Model file for the job. Use its own axes, mm. Face numbers are marked on the shaded views. A direction names the side the tool comes from. Give positions to 0.01 mm unless a question says otherwise; leave off trailing zeros. Order: outer loops, then holes, each group sorted by start corner. A loop starts at its lowest first (then second) coordinate and runs counter-clockwise, first axis right, second up. Notation, with made-up numbers: (-3, 37) -> (13, 37) arc R20 ccw to (13, 76) -> close; hole circle Ø1 at (-19.5, 2). An arc over 180 degrees is marked (long way). Answer in a Markdown table with one row per item. Add a question column.
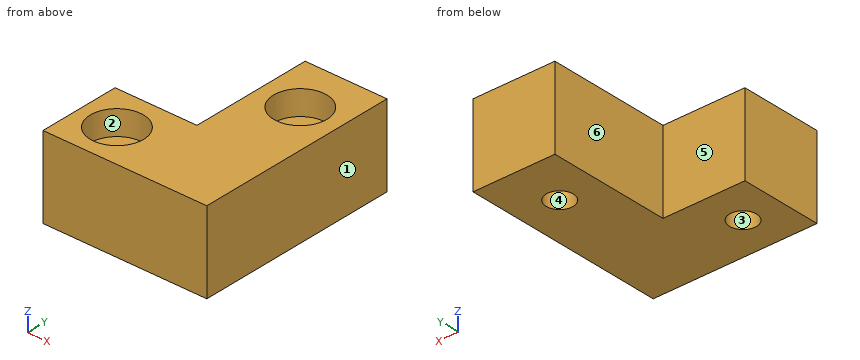
from build123d import *

# Parameters (mm, degrees)
F0_W           = 10
F0_H           = 10
F1_DEPTH       = 25
F2_W           = 10
F2_H           = 10
F3_DEPTH       = 10
F5_D           = 3.3
F5_CBORE_D     = 6.5
F5_CBORE_DEPTH = 3


with BuildPart() as f1:
    # F0 (on Front) → F1 (new body)
    with BuildSketch(Plane.XZ):
        Rectangle(F0_W, F0_H)
    extrude(amount=F1_DEPTH)

    # F2 (on face) → F3 (join)
    with BuildSketch(Plane(origin=(-5, 0, 0), x_dir=(0, -1, 0), z_dir=(-1, 0, 0))):
        with Locations((20, 0)):
            Rectangle(F2_W, F2_H)
    extrude(amount=F3_DEPTH)

    # F5 (through all)
    with Locations(Plane.XY.offset(5)):
        with Locations((0, -6.3472618349), (-10.296119377, -20.085208118)):
            CounterBoreHole(F5_D / 2, F5_CBORE_D / 2, F5_CBORE_DEPTH)


solid = f1.part
Item 1: Saw through at D-D on x = -13. List the corners of the cut face in (y, z).
Item 2: Pin check, flat tips, straight feed: pin 1 Ø12 at (x, y) = (-13, -21.5) entering from +Z; pin 2 Ø2 at (x, y) = (0, -6.35) entering from +Z; pin 3 Ø5 at (x, y) = (0, -6.35) entering from +Z; pin 4 Ø6 at (x, z) = (-9.5, -2.5) entering from +Y. Stop position of each tip, or through.
Item 3: Wall check: line 1 (X direction, y = -20, z = 0.25); line 2 (X direction, y = -12, z = 4.5); line 3 (X direction, y = -7.5, z = -0.25). Give the ranges that are in metal, low to high.
Item 4: Saw through at C-C on y = -19. List the corners of the cut face in (x, z), plus the area to 3 significant figures.
Item 5: Two-plate mould, pull along X, no slides. Class the marked faces 3, 4, 5 and 6: pulls with the +X half, pulls with the -X half, needs draft (parallel to the pull), parting line crosses it, or undercut.
Item 6: Which spindle directions (+Z, -Z, +X, -X, +Y, -Y) get a long thin tool onto all of the face, cutting with end or side? Do the marked faces 1 and 2. Say none if no direction does.
Item 7: Saw through at B-B on z = -2.75. List the corners of the cut face in (x, y).
Item 8: Saw through at A-A on x = 0. List the corners of the cut face in (y, z).
Evaluation:
| question | item | result |
|---|---|---|
| 1 | outline | (-25, -5) -> (-15, -5) -> (-15, 5) -> (-18.28, 5) -> (-18.28, 2) -> (-21.89, 2) -> (-21.89, 5) -> (-25, 5) -> close |
| 2 | pin 1 | stops at z = 5 |
| 2 | pin 2 | passes through |
| 2 | pin 3 | stops at z = 2 |
| 2 | pin 4 | stops at y = -15 |
| 3 | line 1 | x = -15 to -11.94, -8.65 to 5 |
| 3 | line 2 | x = -5 to 5 |
| 3 | line 3 | x = -5 to -1.18, 1.18 to 5 |
| 4 | outline | (-15, -5) -> (-11.54, -5) -> (-11.54, 2) -> (-13.36, 2) -> (-13.36, 5) -> (-15, 5) -> close; (-9.05, -5) -> (5, -5) -> (5, 5) -> (-7.23, 5) -> (-7.23, 2) -> (-9.05, 2) -> close |
| 4 | area | 164 mm2 |
| 5 | face 3 | undercut |
| 5 | face 4 | undercut |
| 5 | face 5 | needs draft |
| 5 | face 6 | pulls with the -X half |
| 6 | face 1 | +Z, -Z, +X, +Y, -Y |
| 6 | face 2 | +Z |
| 7 | outline | (-15, -25) -> (5, -25) -> (5, 0) -> (-5, 0) -> (-5, -15) -> (-15, -15) -> close; hole circle Ø3.3 at (-10.3, -20.09); hole circle Ø3.3 at (0, -6.35) |
| 8 | outline | (-25, -5) -> (-8, -5) -> (-8, 2) -> (-9.6, 2) -> (-9.6, 5) -> (-25, 5) -> close; (-4.7, -5) -> (0, -5) -> (0, 5) -> (-3.1, 5) -> (-3.1, 2) -> (-4.7, 2) -> close |
